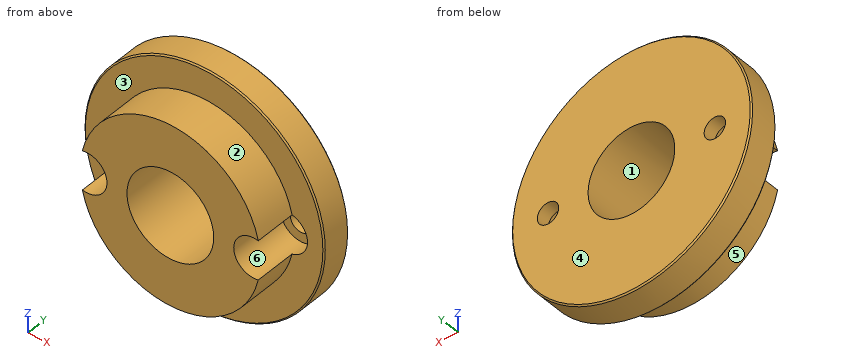
```python
from build123d import *

# Parameters (mm, degrees)
F0_R          = 18
F0_R_2        = 1.6
F0_R_3        = 6.5
F1_DEPTH      = 4.5
F2_SIZE       = 0.2
F3_R          = 6.5
F4_DEPTH      = 6.2
F5_R          = 3
F6_DEPTH      = 2.5
F6_DEPTH_BACK = 6.201


with BuildPart() as f1:
    # F0 (on Front) → F1 (new body)
    with BuildSketch(Plane.XZ):
        Circle(F0_R)
        with Locations((-12.5, 0)):
            Circle(F0_R_2, mode=Mode.SUBTRACT)
        Circle(F0_R_3, mode=Mode.SUBTRACT)
        with Locations((12.5, 0)):
            Circle(F0_R_2, mode=Mode.SUBTRACT)
    extrude(amount=-F1_DEPTH)

    # F2
    f2_edges = [f1.edges().sort_by_distance(p)[0] for p in [
        (-18, 4.5, 0),
        (-18, 0, 0),
    ]]
    chamfer(f2_edges, length=F2_SIZE)

    # F3 (on face) → F4 (join)
    with BuildSketch(Plane.XZ):
        with BuildLine():
            ThreePointArc((-13.4376, 1.2964976822), (-10.9, 0), (-13.4376, -1.2964976822))
            ThreePointArc((-13.4376, -1.2964976822), (0, -13.5), (13.4376, -1.2964976822))
            ThreePointArc((13.4376, -1.2964976822), (10.9, 0), (13.4376, 1.2964976822))
            ThreePointArc((13.4376, 1.2964976822), (0, 13.5), (-13.4376, 1.2964976822))
        make_face()
        Circle(F3_R, mode=Mode.SUBTRACT)
    extrude(amount=F4_DEPTH)

    # F5 (on face) → F6 (cut, two sides)
    with BuildSketch(Plane.XZ) as f6_sk:
        with Locations((-12.5, 0)):
            Circle(F5_R)
        with Locations((12.5, 0)):
            Circle(F5_R)
    extrude(amount=-F6_DEPTH, mode=Mode.SUBTRACT)
    extrude(f6_sk.sketch, amount=F6_DEPTH_BACK, mode=Mode.SUBTRACT)


solid = f1.part
```
Read the model definition and answer for the solid it produces. Units are mm, in the model's axes. Face numbers are marked on the shaded views. A direction names the side the tool comes from. Give positions to 0.01 mm unless a question says otherwise; leave off trailing zeros. Order: outer loops, then holes, each group sorted by start corner. A loop starts at its lowest first (then second) coordinate and runs counter-clockwise, first axis right, second up.
(1) For the marked faces 1, 2 and 3, determine the directions among +Z, -Z, +X, -X, +Y, -Y from which every point of the face is accessible in a straight line to the end or side of a thin tool.
(2) Find section C-C (y = -4.25). Give the vertices of the cut face in (x, z).
(3) Straight lines are drawn through the part: L1, parallel to Y at x = -11.5, z = -7.5; L2, parallel to Z at x = 12, y = -3.5; L3, parallel to Z at x = -12.5, y = -1.5. For each, find the intervals that lie inside material, in ascending order.
(4) Find section D-D (y = 1). Give the vertices of the cut face in (x, z), plus the area to 3 significant figures.
(5) For a pull along X with two mould halves and no side action, classify the marked faces 4, 5 and 6 as released by +X, released by -X, zero draft, split by the parting line, or undercut.
(6) Find section B-B (x = 0). Give the vertices of the cut face in (y, z), plus the area to 3 significant figures.
(7) Given pin 1 (1.9 mm diameter, centred on x = -12.5, z = 0, fed in from -Y); pin 2 (1.5 mm diameter, centred on y = 1, z = 5.5, fed in from -X); pin 3 (3 mm diameter, centred on x = 12.5, z = 0.5, fed in from -Y); pin 4 (1 mm diameter, centred on x = 1, y = -2.5, fed in from -Z), each flat-ended and moving along its own axis, determine where each tip first touches the part or whether it passes through.
(8) Find section A-A (z = 0). Give the vertices of the cut face in (x, y), plus the area to 3 significant figures.
Result sheet:
1. face 1: +Y, -Y
1. face 2: +Z, -Y
1. face 3: -Y
2. outline: (-13.18, -2.92) arc R13.5 ccw to (13.18, -2.92) arc R3 cw (long way) to (13.18, 2.92) arc R13.5 ccw to (-13.18, 2.92) arc R3 cw (long way) to start; hole circle Ø13 at (0, 0)
3. L1: y = 0 to 4.5
3. L2: z = -6.18 to -2.96, 2.96 to 6.18
3. L3: z = -5.1 to -3, 3 to 5.1
4. outline: circle Ø36 at (0, 0); hole circle Ø6 at (-12.5, 0); hole circle Ø13 at (0, 0); hole circle Ø6 at (12.5, 0)
4. area: 829 mm2
5. face 4: zero draft
5. face 5: split by the parting line
5. face 6: undercut
6. outline: (-6.2, -13.5) - (0, -13.5) - (0, -17.8) - (0.2, -18) - (4.3, -18) - (4.5, -17.8) - (4.5, -6.5) - (-6.2, -6.5) - close; (-6.2, 6.5) - (4.5, 6.5) - (4.5, 17.8) - (4.3, 18) - (0.2, 18) - (0, 17.8) - (0, 13.5) - (-6.2, 13.5) - close
6. area: 190 mm2
7. pin 1: passes through
7. pin 2: stops at x = -17.36
7. pin 3: stops at y = 2.5
7. pin 4: stops at z = -13.49
8. outline: (-18, 0.2) - (-17.8, 0) - (-15.5, 0) - (-15.5, 2.5) - (-14.1, 2.5) - (-14.1, 4.5) - (-17.8, 4.5) - (-18, 4.3) - close; (-10.9, 2.5) - (-9.5, 2.5) - (-9.5, -6.2) - (-6.5, -6.2) - (-6.5, 4.5) - (-10.9, 4.5) - close; (6.5, -6.2) - (9.5, -6.2) - (9.5, 2.5) - (10.9, 2.5) - (10.9, 4.5) - (6.5, 4.5) - close; (14.1, 2.5) - (15.5, 2.5) - (15.5, 0) - (17.8, 0) - (18, 0.2) - (18, 4.3) - (17.8, 4.5) - (14.1, 4.5) - close
8. area: 97.8 mm2
